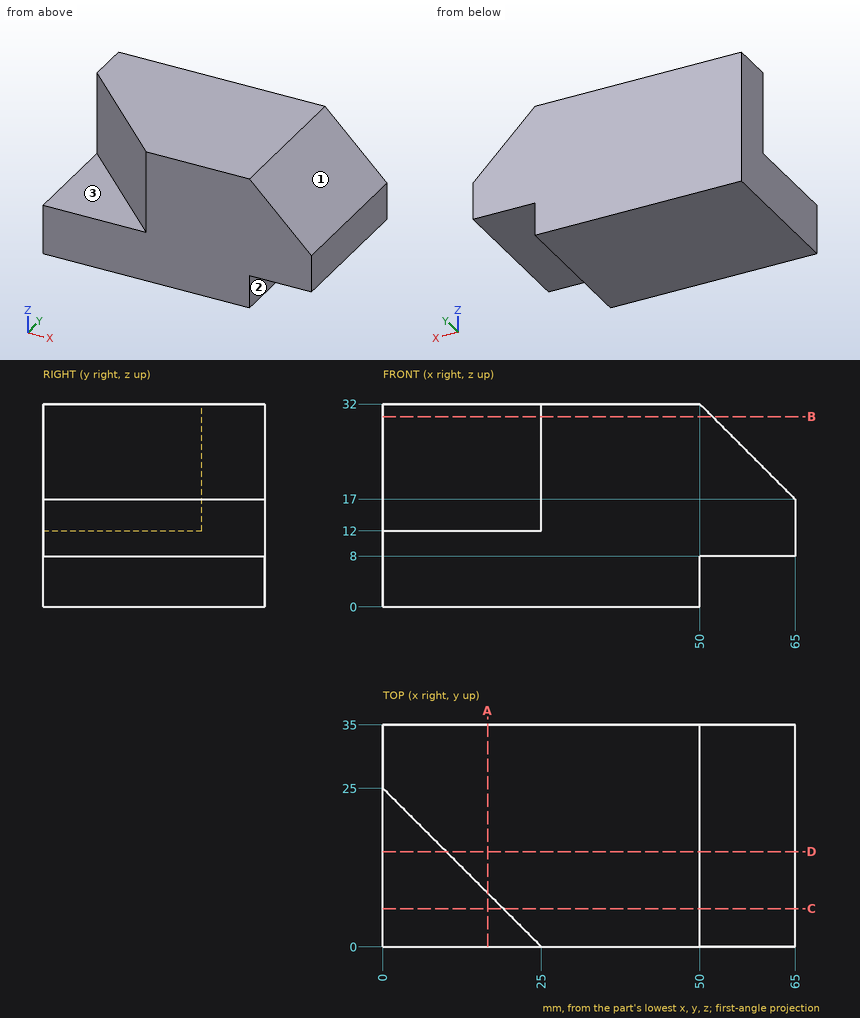
Print and shaded views of the part. All mm, measured from the part's lowest x, y and z. A direction names the side the tool comes from. Give positions to 0.01 mm unless a question says otherwise; leave off trailing zeros. Loops run counter-clockwise (first coordinate to the right, second up) from the corner with the lowest first, then second, coordinate; pieces in that order, holes last. Notation, with made-up numbers: (33, -6.75) -> (62, -6.75) arc R26 ccw to (62, 23.25) -> close; hole circle Ø11 at (57.5, 35.25). An arc over 180 degrees is marked (long way). Use a Markdown table: item, result.
1. Flat gauge pins, fed straight in: pin 1 (4.5 mm diameter, centred on x = 58.5, y = 20.5, fed in from -Z); pin 2 (6.5 mm diameter, centred on y = 26, z = 2.5, fed in from +X); pin 3 (10 mm diameter, centred on y = 11.5, z = 25, fed in from +X). Where does each tip first touch, or does it go through?
Check result:
| item | result |
|---|---|
| pin 1 | stops at z = 8 |
| pin 2 | stops at x = 50 |
| pin 3 | stops at x = 62 |
2. Slice it at B-B (z = 30). List the corners of the cut face in (x, y).
Check result:
| item | result |
|---|---|
| outline | (0, 25) -> (25, 0) -> (52, 0) -> (52, 35) -> (0, 35) -> close |
3. Which spindle directions (+Z, -Z, +X, -X, +Y, -Y) get a long thin tool onto all of the face, cutting with end or side? Do the marked faces 1, 2 and 3. Say none if no direction does.
Check result:
| item | result |
|---|---|
| face 1 | +Z, +X, +Y, -Y |
| face 2 | -Z, +X, +Y, -Y |
| face 3 | +Z, -X, -Y |
4. Slice it at C-C (y = 6). List the corners of the cut face in (x, z).
Check result:
| item | result |
|---|---|
| outline | (0, 0) -> (50, 0) -> (50, 8) -> (65, 8) -> (65, 17) -> (50, 32) -> (19, 32) -> (19, 12) -> (0, 12) -> close |
5. Slice it at A-A (x = 16.5). List the corners of the cut face in (y, z), plus the area to 3 significant figures.
Check result:
| item | result |
|---|---|
| outline | (0, 0) -> (35, 0) -> (35, 32) -> (8.5, 32) -> (8.5, 12) -> (0, 12) -> close |
| area | 950 mm^2 |
6. Slice it at D-D (y = 15). List the corners of the cut face in (x, z).
Check result:
| item | result |
|---|---|
| outline | (0, 0) -> (50, 0) -> (50, 8) -> (65, 8) -> (65, 17) -> (50, 32) -> (10, 32) -> (10, 12) -> (0, 12) -> close |
7. Wall check: L1, parallel to X at y = 17, z = 7; L2, parallel to Z at x = 6, y = 2; L3, parallel to X at y = 8.5, z = 24.5. Give the ranges that are in metal, low to high. Write a range as [from, to].
Check result:
| item | result |
|---|---|
| L1 | x = [0, 50] |
| L2 | z = [0, 12] |
| L3 | x = [16.5, 57.5] |
